from build123d import *

# Parameters (mm, degrees)
F0_R     = 6.35
F1_DEPTH = 3.175


with BuildPart() as f1:
    # F0 (on Top) → F1 (new body)
    with BuildSketch(Plane.XY):
        with BuildLine():
            Line((50.245686, -33.959337), (59.226047, -24.978976))
            ThreePointArc((59.226047, -24.978976), (61.085919, -20.48891), (59.226135, -15.998808))
            Line((59.226135, -15.998808), (20.675575, 22.553266))
            ThreePointArc((20.675575, 22.553266), (18.615456, 23.929837), (16.185359, 24.413226))
            Line((16.185359, 24.413226), (-38.334312, 24.413226))
            ThreePointArc((-38.334312, 24.413226), (-42.82444, 22.553354), (-44.684312, 18.063226))
            Line((-44.684312, 18.063226), (-44.684312, 11.716822))
            Line((-44.684312, 11.716822), (-44.684312, 5.363226))
            ThreePointArc((-44.684312, 5.363226), (-42.82444, 0.873098), (-38.334312, -0.986774))
            Line((-38.334312, -0.986774), (3.558176, -0.986774))
            ThreePointArc((3.558176, -0.986774), (7.932227, -1.856822), (11.640375, -4.334512))
            Line((11.640375, -4.334512), (41.265447, -33.959355))
            ThreePointArc((41.265447, -33.959355), (45.75557, -35.819209), (50.245686, -33.959337))
        make_face()
        with Locations((-34.088506, 11.716822)):
            Circle(F0_R, mode=Mode.SUBTRACT)
        with Locations((-2.338506, 11.716822)):
            Circle(F0_R, mode=Mode.SUBTRACT)
    extrude(amount=F1_DEPTH)


solid = f1.part
Can you work these out from the model? Positions are in its coordinate system, mm. A direction names the side the tool comes from. Round coordinates to 2 decimals unless told otherwise and drop trailing zeros. Loops run counter-clockwise (first coordinate to the right, second up) from the corner with the lowest first, then second, coordinate; pieces in that order, holes last. Notation, with made-up numbers: (19, 4.25) - (73, 4.25) arc R15 cw to (73, 16.25) - close; hole circle Ø6 at (22.25, 11.25). An arc over 180 degrees is marked (long way). Answer in a Markdown table with one row per item. Add a question column.
Q1. Which directions (+Z, -Z, +X, -X, +Y, -Y) give clear straight access to the entire face, cutting with the end or side of a thin tool? Please do faces 4 (the flat face through (-18, -0.987, 2)), 5 (the cylindrical face through (18.648, 23.916, 1.565)).
Q2. I want a section at B-B on z = 0.55. List the corners of the cut face in (x, y) for me, and give its area (3 significant figures).
Q3. I want a section at A-A on y = 10. List the corners of the cut face in (x, z) for me (3 decimals).
Q4. I need wall thicknesses on L1, parallel to Y at x = -20, z = 2.7; L2, parallel to Y at x = -2.5, z = 1.15; L3, parallel to X at y = 6, z = 0.5. Which ranges of each line are inside material? Lowest first, please.
Q5. I want a section at D-D on y = -23. List the corners of the cut face in (x, z) for me (3 decimals).
Q6. I want a section at C-C on x = -16. List the corners of the cut face in (y, z) for me (3 decimals), and give its area (3 significant figures).
Q7. We'd pull the mould along X, two halves only. Please class faces 1 (the cylindrical face through (-3.72, 5.52, 1.57)), 2 (the flat face through (-11, 24.413, 2)), 3 (the flat face through (40.22, 3.01, 1.57)): pulls with the +X half, pulls with the -X half, needs draft (parallel to the pull), parting line crosses it, or undercut.
Q8. For pin 1 Ø1.6 at (x, z) = (-26.5, 1) entering from -Y, with a flat end and sliding along its axis, tell me the tip position at first contact or that it passes through.
A:
| question | item | result |
|---|---|---|
| 1 | face 4 | +Z, -Z, -X, -Y |
| 1 | face 5 | +Z, -Z, +X, +Y |
| 2 | outline | (-44.68, 5.36) arc R6.35 ccw to (-38.33, -0.99) - (3.56, -0.99) arc R11.43 cw to (11.64, -4.33) - (41.27, -33.96) arc R6.35 ccw to (50.25, -33.96) - (59.23, -24.98) arc R6.35 ccw to (59.23, -16) - (20.68, 22.55) arc R6.35 ccw to (16.19, 24.41) - (-38.33, 24.41) arc R6.35 ccw to (-44.68, 18.06) - close; hole circle Ø12.7 at (-34.09, 11.72); hole circle Ø12.7 at (-2.34, 11.72) |
| 2 | area | 2,670 mm^2 |
| 3 | outline | (-44.684, 0) - (-40.202, 0) - (-40.202, 3.175) - (-44.684, 3.175) - close; (-27.975, 0) - (-8.452, 0) - (-8.452, 3.175) - (-27.975, 3.175) - close; (3.775, 0) - (33.228, 0) - (33.228, 3.175) - (3.775, 3.175) - close |
| 4 | L1 | -0.99 to 24.41 |
| 4 | L2 | -0.99 to 5.37, 18.06 to 24.41 |
| 4 | L3 | -44.68 to -36.85, -31.32 to -5.1, 0.43 to 37.23 |
| 5 | outline | (30.306, 0) - (60.568, 0) - (60.568, 3.175) - (30.306, 3.175) - close |
| 6 | outline | (-0.987, 0) - (24.413, 0) - (24.413, 3.175) - (-0.987, 3.175) - close |
| 6 | area | 80.6 mm^2 |
| 7 | face 1 | undercut |
| 7 | face 2 | needs draft |
| 7 | face 3 | pulls with the +X half |
| 8 | pin 1 | y = -0.99 |
